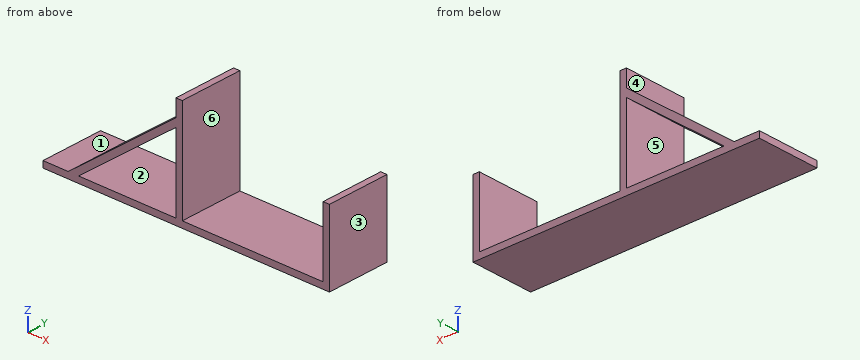
from build123d import *

# Parameters (mm, degrees)
BOSS_EXTRUDE2_DEPTH = 30
CUT_EXTRUDE1_DEPTH  = 30


with BuildPart() as part:
    # Sketch1 → Boss-Extrude2 (new body)
    with BuildSketch(Plane(origin=(0, 10, 0), x_dir=(1, 0, 0), z_dir=(0, 1, 0))):
        Polygon((71.5, -22), (71.5, 13), (-64.73475383, 13), (-64.73475383, 10), (-52.73475383, 10), (-1.5, -30), (-1.5, -38), (1.5, -38), (1.5, 10), (68.5, 10), (68.5, -22), align=None)
    extrude(amount=BOSS_EXTRUDE2_DEPTH)

    # Sketch4 → Cut-Extrude1 (cut)
    with BuildSketch(Plane.XZ.offset(-10)):
        Polygon((-47.85975383, -10), (-1.5, 26.193989716), (-1.5, -10), align=None)
    extrude(amount=-CUT_EXTRUDE1_DEPTH, mode=Mode.SUBTRACT)


solid = part.part
Could you check a few things on this model? Use its own coordinates, in mm. Face numbers are marked on the shaded views. A direction names the side the tool comes from. Give positions to 0.01 mm unless a question says otherwise; leave off trailing zeros. Write each loop counter-clockwise with the first axis right and the second up, starting at its lowest first coordinate (ties: lowest second). Pieces come first, ordered by that corner, then holes. Notation, with made-up numbers: (41.5, 70.5) -> (56.5, 70.5) arc R14 cw to (56.5, 77.5) -> close; hole circle Ø11 at (-40, 68). An arc over 180 degrees is marked (long way). Answer as CSV lines item,"result". Start each with the question number.
(1) I'm going to push flat-ended pins straight in: pin 1 Ø15 at (y, z) = (23, 9) entering from -X; pin 2 Ø9 at (y, z) = (28, 9) entering from -X; pin 3 Ø2 at (y, z) = (26, 16) entering from -X. Where does each tip first touch, or does it pass through?
(2) If we section it at B-B, the plane y = 13.75: Write out the boundary of the cut face in (x, z).
(3) If we section it at D-D, the plane z = 35: Write out the boundary of the cut face in (x, y).
(4) Which directions (+Z, -Z, +X, -X, +Y, -Y) give clear straight access to the entire face, cutting with the end or side of a thin tool? Please do the marked faces 4, 5 and 6.
(5) Please list where these lines run through material, in increasing order: line 1 (X direction, y = 22, z = -4); line 2 (X direction, y = 12.5, z = 6.5); line 3 (Z direction, x = 18.5, y = 36).
(6) If we mould it in two halves opening along Z, with no side actions, what happens to the marked faces 1, 2 and 3? For each: +Z half, -Z half, draft (parallel to the pull), parting line (faces both ways), or undercut.
(7) If we section it at C-C, the plane x = -29.5: Write out the boundary of the cut face in (y, z).
(8) If we section it at A-A, the plane z = 17.5: Write out the boundary of the cut face in (x, y).
Answer list:
1,pin 1,"x = -38"
1,pin 2,"x = -34.16"
1,pin 3,"x = -20.71"
2,outline,"(-64.73, -13) -> (71.5, -13) -> (71.5, 22) -> (68.5, 22) -> (68.5, -10) -> (1.5, -10) -> (1.5, 38) -> (-1.5, 38) -> (-1.5, 30) -> (-52.73, -10) -> (-64.73, -10) -> close; hole (-47.86, -10) -> (-1.5, -10) -> (-1.5, 26.19) -> close"
3,outline,"(-1.5, 10) -> (1.5, 10) -> (1.5, 40) -> (-1.5, 40) -> close"
4,face 4,"+Z, -X, +Y, -Y"
4,face 5,"+Y, -Y"
4,face 6,"+Z, +Y, -Y"
5,line 1,"-45.05 to -40.17, -1.5 to 1.5, 68.5 to 71.5"
5,line 2,"-31.6 to -26.73, -1.5 to 1.5, 68.5 to 71.5"
5,line 3,"-13 to -10"
6,face 1,"+Z half"
6,face 2,"undercut"
6,face 3,"draft"
7,outline,"(10, -13) -> (40, -13) -> (40, -10) -> (10, -10) -> close; (10, 4.33) -> (40, 4.33) -> (40, 8.14) -> (10, 8.14) -> close"
8,outline,"(-17.51, 10) -> (-12.64, 10) -> (-12.64, 40) -> (-17.51, 40) -> close; (-1.5, 10) -> (1.5, 10) -> (1.5, 40) -> (-1.5, 40) -> close; (68.5, 10) -> (71.5, 10) -> (71.5, 40) -> (68.5, 40) -> close"
